Could you check a few things on this model? Use its own coordinates, in mm. A direction names the side the tool comes from. Coordinates: 2 decimals unless noted, no trailing zeros. Order: outer loops, then holes, each group sorted by start corner. A loop starts at its lowest first (then second) coordinate and runs counter-clockwise, first axis right, second up. Notation, with made-up numbers: (53.25, 76.25) - (58.25, 76.25) arc R26 cw to (58.25, 101.25) - close; hole circle Ø4 at (5, 64.5). An arc over 180 degrees is marked (long way). One line per item, written item: value.
from build123d import *

# Parameters (mm, degrees)
F0_W     = 12.7
F0_H     = 38.1
F1_DEPTH = 226.6
F3_D     = 3.7973
F3_DEPTH = 15.875
F3_TIP   = 1.1408240143
F5_D     = 3.7973
F5_DEPTH = 15.875
F5_TIP   = 1.1408240143
F7_D     = 5.1054


with BuildPart() as f1:
    # F0 (on Front) → F1 (new body)
    with BuildSketch(Plane.XZ):
        with Locations((6.35, 19.05)):
            Rectangle(F0_W, F0_H)
    extrude(amount=F1_DEPTH)

    # F3
    with Locations(Plane.XZ.offset(226.6)):
        with Locations((6.35, 31.75), (6.35, 6.35)):
            Hole(F3_D / 2, depth=F3_DEPTH)
            with Locations((0, 0, -(F3_DEPTH + F3_TIP / 2))):  # 118° drill point
                Cone(0, F3_D / 2, F3_TIP, mode=Mode.SUBTRACT)

    # F5
    with Locations(Plane(origin=(0, 0, 0), x_dir=(-1, 0, 0), z_dir=(0, 1, 0))):
        with Locations((-6.35, 31.75), (-6.35, 6.35)):
            Hole(F5_D / 2, depth=F5_DEPTH)
            with Locations((0, 0, -(F5_DEPTH + F5_TIP / 2))):  # 118° drill point
                Cone(0, F5_D / 2, F5_TIP, mode=Mode.SUBTRACT)

    # F7 (through all)
    with Locations(Plane(origin=(0, 0, 0), x_dir=(1, 0, 0), z_dir=(0, 0, -1))):
        with Locations((6.35, 25.4), (6.35, 201.2)):
            Hole(F7_D / 2)


solid = f1.part
Item 1: I want a section at A-A on y = -25.4. Please give me the cut outline in (x, z), then the cut area to 3 significant figures.
Conclusion:
outline: (0, 0) - (3.8, 0) - (3.8, 38.1) - (0, 38.1) - close; (8.9, 0) - (12.7, 0) - (12.7, 38.1) - (8.9, 38.1) - close
area: 289 mm²
Item 2: If I drill on probe 1 along Z at (x, y) = (6.35, -4.25); probe 2 along Y at (x, z) = (6.35, 13); probe 3 along X at (y, z) = (-5.5, 31.75), over which ranges is the centre line in solid material (lowest first)?
Conclusion:
probe 1: 0 to 4.45, 8.25 to 29.85, 33.65 to 38.1
probe 2: -226.6 to -203.75, -198.65 to -27.95, -22.85 to 0
probe 3: 0 to 4.45, 8.25 to 12.7
Item 3: Thinking about a two-plate mould opening in Z: for faces 4 (the face through (6, -112, 0)), 5 (the face through (6, 0, 19)), 6 (the face through (6.597, -218.551, 33.632)), which applies, pulls with the +Z half, pulls with the -Z half, needs draft (parallel to the pull), parting line crosses it, or undercut?
Conclusion:
face 4: pulls with the -Z half
face 5: needs draft
face 6: undercut
Item 4: For faces 1 (the face through (6.103, -8.049, 33.632)), 2 (the face through (6, -112, 38.1)), 3 (the face through (7.857, -218.551, 5.195)), which set-ups out of +Z, -Z, +X, -X, +Y, -Y let a thin tool reach every point of the face, with its end or its side?
Conclusion:
face 1: +Y
face 2: +Z, +X, -X, +Y, -Y
face 3: -Y
Item 5: I'm going to push a flat-ended pin straight in: pin 1 Ø2.5 at (x, z) = (6.35, 31.75) entering from -Y. Where does the tip first touch, or does it pass through?
Conclusion:
pin 1: y = -210.34
